Can you work these out from the model? Positions are in its coordinate system, mm. Coordinates: 2 decimals unless noted, no trailing zeros. Write each loop counter-clockwise with the first axis right and the second up, starting at its lowest first coordinate (ties: lowest second). Pieces come first, ordered by that corner, then holes. Notation, with made-up numbers: (4.25, -6) - (27.25, -6) arc R16 ccw to (27.25, -2) - close; hole circle Ø8 at (15, 81.25). An arc over 180 degrees is marked (long way). Use one line per item in the form item = value. Start each with the question number.
(1) For pin 1 Ø1.5 at (x, z) = (25.5, -0.5) entering from -Y (3 decimals); pin 2 Ø5.5 at (x, y) = (0, -25.4) entering from -Z, each with a flat end and sliding along its axis, tell me the tip position at first contact or that it passes through.
(2) If we section it at D-D on x = 47.5: Please give me the cut outline in (y, z) (3 decimals).
(3) If we section it at C-C on y = 16.5: Please give me the cut outline in (x, z) (3 decimals), then the cut area to 4 significant figures.
(4) If we section it at A-A on z = 0.45: Give the number of separate pieces and of enclosed holes in the cut face, then the cut area to 3 significant figures.
(5) If I drill on probe 1 along Y at (x, z) = (12.7, 0.1) (3 decimals); probe 2 along Y at (x, z) = (21, 0.8) (3 decimals); probe 3 along X at (y, z) = (16, -0.85) (3 decimals), over which ranges is the centre line in solid material (lowest first)? Write a range as from..to.
(6) If we section it at B-B on x = 12.7: Please give me the cut outline in (y, z) (3 decimals), then the cut area to 3 significant figures.
```python
from build123d import *

# Parameters (mm, degrees)
SKETCH1_R           = 2.075
BOSS_EXTRUDE2_DEPTH = 1.5
FILLET2_R           = 3


with BuildPart() as part:
    # Sketch1 → Boss-Extrude2 (new, symmetric)
    with BuildSketch(Plane.XY):
        with BuildLine():
            Line((-5.075, 38.1), (-5.075, -63.5))
            ThreePointArc((-5.075, -63.5), (0, -68.575), (5.075, -63.5))
            Line((5.075, -63.5), (5.075, -10.075))
            Line((5.075, -10.075), (50.8, -10.075))
            ThreePointArc((50.8, -10.075), (60.875, 0), (50.8, 10.075))
            Line((50.8, 10.075), (5.075, 10.075))
            Line((5.075, 10.075), (5.075, 38.1))
            ThreePointArc((5.075, 38.1), (0, 43.175), (-5.075, 38.1))
        make_face()
        Circle(SKETCH1_R, mode=Mode.SUBTRACT)
        with Locations((12.7, 0)):
            Circle(SKETCH1_R, mode=Mode.SUBTRACT)
        with Locations((25.4, 0)):
            Circle(SKETCH1_R, mode=Mode.SUBTRACT)
        with Locations((38.1, 0)):
            Circle(SKETCH1_R, mode=Mode.SUBTRACT)
        with Locations((50.8, 0)):
            Circle(SKETCH1_R, mode=Mode.SUBTRACT)
        with Locations((0, 12.7)):
            Circle(SKETCH1_R, mode=Mode.SUBTRACT)
        with Locations((0, 25.4)):
            Circle(SKETCH1_R, mode=Mode.SUBTRACT)
        with Locations((0, 38.1)):
            Circle(SKETCH1_R, mode=Mode.SUBTRACT)
        with Locations((0, -12.7)):
            Circle(SKETCH1_R, mode=Mode.SUBTRACT)
        with Locations((0, -25.4)):
            Circle(SKETCH1_R, mode=Mode.SUBTRACT)
        with Locations((0, -38.1)):
            Circle(SKETCH1_R, mode=Mode.SUBTRACT)
        with Locations((0, -50.8)):
            Circle(SKETCH1_R, mode=Mode.SUBTRACT)
        with Locations((0, -63.5)):
            Circle(SKETCH1_R, mode=Mode.SUBTRACT)
    extrude(amount=BOSS_EXTRUDE2_DEPTH, both=True)

    # Fillet2
    fillet2_edges = [part.edges().sort_by_distance(p)[0] for p in [
        (5.075, 10.075, 0),
        (5.075, -10.075, 0),
    ]]
    fillet(fillet2_edges, radius=FILLET2_R)


solid = part.part
```
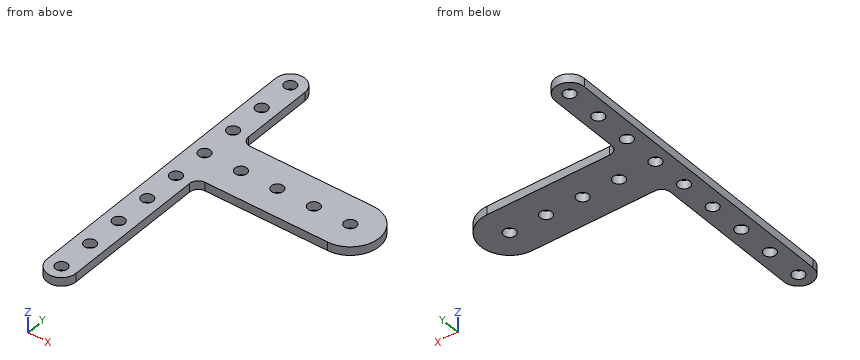
Reported:
q1.pin_1 = -10.075
q1.pin_2 = -1.5
q2.outline = (-10.075, -1.5) - (10.075, -1.5) - (10.075, 1.5) - (-10.075, 1.5) - close
q3.outline = (-5.075, -1.5) - (5.075, -1.5) - (5.075, 1.5) - (-5.075, 1.5) - close
q3.area = 30.45 mm2
q4.separate_pieces = 1
q4.enclosed_holes = 13
q4.area = 2,020 mm2
q5.probe_1 = -10.075..-2.075, 2.075..10.075
q5.probe_2 = -10.075..10.075
q5.probe_3 = -5.075..5.075
q6.outline = (-10.075, -1.5) - (-2.075, -1.5) - (-2.075, 1.5) - (-10.075, 1.5) - close; (2.075, -1.5) - (10.075, -1.5) - (10.075, 1.5) - (2.075, 1.5) - close
q6.area = 48.0 mm2
